Check sheet for the modelled part. Datum: model origin and axes. Units: mm. A direction names the side the tool comes from. Round coordinates to 2 decimals unless told otherwise and drop trailing zeros. Write each loop counter-clockwise with the first axis right and the second up, starting at its lowest first coordinate (ties: lowest second). Pieces come first, ordered by that corner, then holes.
Item 1: Cross-section at B-B on x = -4. Enter the section's corners in (y, z), plus the area to 3 significant figures.
Item 2: Go/stop test with flat-tipped pins: pin 1 Ø1.5 at (x, z) = (-5.5, 3.5) entering from -Y; pin 2 Ø2 at (x, z) = (-3, 3.5) entering from -Y; pin 3 Ø13 at (x, y) = (7.5, -4) entering from -Z. Record where each tip stops, or that it passes through.
Item 3: Cross-section at C-C on y = 12. Enter the section's corners in (x, z).
Item 4: Cross-section at A-A on z = 1.2. Enter the section's corners in (x, y), plus the area to 3 significant figures.
Item 5: Cross-section at D-D on z = 3.6. Enter the section's corners in (x, y).
Item 6: Material ranges on line 1 (X direction, y = 0.5, z = 2.2); line 2 (Z direction, x = 11, y = 4); line 3 (Y direction, x = 12, z = 1.6), recorded low to high.
Item 7: Tool access check on faces 5 (the cylindrical face through (12.78, -13.03, 1.48)), 6 (the flat face through (2, -18.6, 1.5)), 7 (the flat face through (14, 12, 0)), 8 (the flat face through (0, 0, 5)), 9 (the flat face through (19, 0, 1)). Record the directions out of +Z, -Z, +X, -X, +Y, -Y that give a thin tool (end or side, any length) a straight path to the whole face; none if there is none.
Item 8: Release check for a two-part mould opening along X. For faces 1 (the flat face through (0, -19, 1)), 2 (the cylindrical face through (14.43, 12.74, 1.48)), 3 (the cylindrical face through (-13.46, 13.76, 1.48)), 4 (the flat face through (-18.6, -2, 1.5)) record: +X half, -X half, draft (parallel to the pull), parting line (faces both ways), or undercut.
from build123d import *

# Parameters (mm, degrees)
SCHIZZO1_R                   = 19.25
SCHIZZO1_R_2                 = 18.25
ESTRUSIONE_ESTRUSIONE1_DEPTH = 3
SCHIZZO2_R                   = 22
ESTRUSIONE_ESTRUSIONE2_DEPTH = 2
TAGLIO_ESTRUSIONE1_DEPTH     = 3


with BuildPart() as part:
    # Schizzo1 → Estrusione-Estrusione1 (new body)
    with BuildSketch(Plane.XY):
        Circle(SCHIZZO1_R)
        Circle(SCHIZZO1_R_2, mode=Mode.SUBTRACT)
    extrude(amount=ESTRUSIONE_ESTRUSIONE1_DEPTH)

    # Schizzo2 → Estrusione-Estrusione2 (add)
    with BuildSketch(Plane.XY.offset(3)):
        Circle(SCHIZZO2_R)
    extrude(amount=ESTRUSIONE_ESTRUSIONE2_DEPTH)

    # Schizzo3 → Taglio-Estrusione1 (cut)
    with BuildSketch(Plane(origin=(0, 0, 0), x_dir=(-1, 0, 0), z_dir=(0, 0, -1))):
        with BuildLine():
            Line((0, 18.25), (0, 19.25))
            ThreePointArc((0, 19.25), (-1.001355713, 19.223937857), (-2, 19.145821999))
            Line((-2, 19.145821999), (-2, 18.140079934))
            ThreePointArc((-2, 18.140079934), (-1.001509164, 18.222499263), (0, 18.25))
        make_face()
        with BuildLine():
            Line((-18.25, 0), (-19.25, 0))
            ThreePointArc((-19.25, 0), (-19.223937857, -1.001355713), (-19.145821999, -2))
            Line((-19.145821999, -2), (-18.140079934, -2))
            ThreePointArc((-18.140079934, -2), (-18.222499263, -1.001509164), (-18.25, 0))
        make_face()
        with BuildLine():
            ThreePointArc((-2, -19.145821999), (-1.001355713, -19.223937857), (0, -19.25))
            Line((0, -19.25), (0, -18.25))
            ThreePointArc((0, -18.25), (-1.001509164, -18.222499263), (-2, -18.140079934))
            Line((-2, -18.140079934), (-2, -19.145821999))
        make_face()
        with BuildLine():
            ThreePointArc((19.145821999, -2), (19.223937857, -1.001355713), (19.25, 0))
            Line((19.25, 0), (18.25, 0))
            ThreePointArc((18.25, 0), (18.222499263, -1.001509164), (18.140079934, -2))
            Line((18.140079934, -2), (19.145821999, -2))
        make_face()
    extrude(amount=-TAGLIO_ESTRUSIONE1_DEPTH, mode=Mode.SUBTRACT)


solid = part.part
Response values:
1. outline: (-21.63, 3) - (-18.83, 3) - (-18.83, 0) - (-17.81, 0) - (-17.81, 3) - (17.81, 3) - (17.81, 0) - (18.83, 0) - (18.83, 3) - (21.63, 3) - (21.63, 5) - (-21.63, 5) - close
1. area: 92.7 mm2
2. pin 1: stops at y = -21.48
2. pin 2: stops at y = -21.91
2. pin 3: stops at z = 3
3. outline: (-18.44, 3) - (-15.05, 3) - (-15.05, 0) - (-13.75, 0) - (-13.75, 3) - (13.75, 3) - (13.75, 0) - (15.05, 0) - (15.05, 3) - (18.44, 3) - (18.44, 5) - (-18.44, 5) - close
4. outline: (-19.25, 0) - (-18.25, 0) arc R18.25 cw to (0, 18.25) - (0, 19.25) arc R19.25 ccw to start; (-19.15, -2) arc R19.25 ccw to (0, -19.25) - (0, -18.25) arc R18.25 cw to (-18.14, -2) - close; (2, -19.15) arc R19.25 ccw to (19.15, -2) - (18.14, -2) arc R18.25 cw to (2, -18.14) - close; (2, 18.14) arc R18.25 cw to (18.25, 0) - (19.25, 0) arc R19.25 ccw to (2, 19.15) - close
4. area: 110 mm2
5. outline: circle Ø44 at (0, 0)
6. line 1: x = -19.24 to -18.24, 18.24 to 19.24
6. line 2: z = 3 to 5
6. line 3: y = -15.05 to -13.75, 13.75 to 15.05
7. face 5: -Z
7. face 6: -Z, +Y, -Y
7. face 7: -Z, +X, -X, +Y, -Y
7. face 8: +Z, +X, -X, +Y, -Y
7. face 9: -Z, +X, -X
8. face 1: undercut
8. face 2: +X half
8. face 3: -X half
8. face 4: draft
